from build123d import *

# Parameters (mm, degrees)
F0_W     = 156
F0_H     = 70
F0_H_2   = 80
F0_H_3   = 20
F1_DEPTH = 50
F2_W     = 150
F2_H     = 17.901978
F2_H_2   = 71.477221
F2_H_3   = 62.391793
F3_DEPTH = 70
F4_W     = 150
F4_H     = 44
F5_DEPTH = 200
F6_W     = 44
F6_H     = 17.90198
F6_H_2   = 71.47722
F6_H_3   = 62.39179
F7_DEPTH = 200


with BuildPart() as f1:
    # F0 (on Front) → F1 (new body)
    with BuildSketch(Plane.XZ):
        with Locations((3.490141, 35)):
            Rectangle(F0_W, F0_H)
        with Locations((3.490141, -40)):
            Rectangle(F0_W, F0_H_2)
        with Locations((3.490141, -90)):
            Rectangle(F0_W, F0_H_3)
    extrude(amount=-F1_DEPTH)

    # F2 (on face) → F3 (cut)
    with BuildSketch(Plane(origin=(0, 50, 0), x_dir=(-1, 0, 0), z_dir=(0, 1, 0))):
        with Locations((-3.490141, -91.049011)):
            Rectangle(F2_W, F2_H)
        with Locations((-3.490141, -39.823143)):
            Rectangle(F2_W, F2_H_2)
        with Locations((-3.490141, 34.804103)):
            Rectangle(F2_W, F2_H_3)
    extrude(amount=-F3_DEPTH, mode=Mode.SUBTRACT)

    # F4 (on face) → F5 (cut)
    with BuildSketch(Plane.XY.offset(70)):
        with Locations((3.490141, 25)):
            Rectangle(F4_W, F4_H)
    extrude(amount=-F5_DEPTH, mode=Mode.SUBTRACT)

    # F6 (on face) → F7 (cut)
    with BuildSketch(Plane.YZ.offset(81.490141)):
        with Locations((25, -91.04901)):
            Rectangle(F6_W, F6_H)
        with Locations((25, -42.506896)):
            Rectangle(F6_W, F6_H_2)
        with Locations((25, 34.174311)):
            Rectangle(F6_W, F6_H_3)
    extrude(amount=-F7_DEPTH, mode=Mode.SUBTRACT)


solid = f1.part
Part model, mm, in its own coordinate system. A direction names the side the tool comes from. Give positions to 0.01 mm unless a question says otherwise; leave off trailing zeros. Order: outer loops, then holes, each group sorted by start corner. A loop starts at its lowest first (then second) coordinate and runs counter-clockwise, first axis right, second up. Notation, with made-up numbers: (53.5, 16.5) - (91.5, 16.5) arc R12 cw to (91.5, 32.5) - close; hole circle Ø5 at (-25.75, 35.5). An arc over 180 degrees is marked (long way). Use a Markdown table: item, result.
1) Saw through at A-A on x = 40. List the corners of the cut face in (y, z), plus the area to 3 significant figures.
Checked values:
| item | result |
|---|---|
| outline | (0, -82.1) - (3, -82.1) - (3, -75.56) - (0, -75.56) - close; (0, -4.08) - (3, -4.08) - (3, 3.61) - (0, 3.61) - close; (0, 66) - (3, 66) - (3, 70) - (0, 70) - close; (47, -82.1) - (50, -82.1) - (50, -75.56) - (47, -75.56) - close; (47, -4.08) - (50, -4.08) - (50, 3.61) - (47, 3.61) - close; (47, 66) - (50, 66) - (50, 70) - (47, 70) - close |
| area | 109 mm² |
2) 3-axis set-ups, long thin cutter, end or side, ignore diameter. For faces 1 (the flat face through (2, 47, 68)), 2 (the flat face through (78.49, 23, 66)), 3 (the flat face through (-20, 0, -2)): which of +Z, -Z, +X, -X, +Y, -Y reach the whole face in a straight line?
Checked values:
| item | result |
|---|---|
| face 1 | +Z, -Z |
| face 2 | none |
| face 3 | +Z, -Z, +X, -X, -Y |
3) Two-plate mould, pull along Z, no slides. Class faces 4 (the flat face through (-14.2, 2.7, 70)), 5 (the flat face through (-71.51, 25, -4)), 6 (the flat face through (81.49, 25, -3)): +Z half, -Z half, draft (parallel to the pull), parting line (faces both ways), or undercut.
Checked values:
| item | result |
|---|---|
| face 4 | +Z half |
| face 5 | undercut |
| face 6 | draft |
4) Flat gauge pins, fed straight in: P1, Ø3.5, axis at x = 80, y = 33, coming from the -Z side; P2, Ø15, axis at y = 35, z = -23.5, coming from the -X side. Where does each tip first touch, or does it go through?
Checked values:
| item | result |
|---|---|
| P1 | z = -82.1 |
| P2 | through |
5) Probe L1, parallel to X at y = 33.5, z = -6; L2, parallel to Y at x = -30.5, z = -79. List the from-to ranges inside material, lowest first. Write a range as from..to.
Checked values:
| item | result |
|---|---|
| L1 | -74.51..-71.51, 78.49..81.49 |
| L2 | 0..3, 47..50 |
6) Saw through at C-C on z = -32.5. List the corners of the cut face in (x, y), plus the area to 3 significant figures.
Checked values:
| item | result |
|---|---|
| outline | (-74.51, 0) - (-71.51, 0) - (-71.51, 3) - (-74.51, 3) - close; (-74.51, 47) - (-71.51, 47) - (-71.51, 50) - (-74.51, 50) - close; (78.49, 0) - (81.49, 0) - (81.49, 3) - (78.49, 3) - close; (78.49, 47) - (81.49, 47) - (81.49, 50) - (78.49, 50) - close |
| area | 36.0 mm² |
7) Saw through at B-B on y = 21. List the corners of the cut face in (x, z).
Checked values:
| item | result |
|---|---|
| outline | (-74.51, -82.1) - (-71.51, -82.1) - (-71.51, -78.25) - (-74.51, -78.25) - close; (-74.51, -6.77) - (-71.51, -6.77) - (-71.51, 2.98) - (-74.51, 2.98) - close; (-74.51, 65.37) - (-71.51, 65.37) - (-71.51, 70) - (-74.51, 70) - close; (78.49, -82.1) - (81.49, -82.1) - (81.49, -78.25) - (78.49, -78.25) - close; (78.49, -6.77) - (81.49, -6.77) - (81.49, 2.98) - (78.49, 2.98) - close; (78.49, 65.37) - (81.49, 65.37) - (81.49, 70) - (78.49, 70) - close |
